Verification items for this drawing (mm, ordinates from the low corner). A direction names the side the tool comes from. Coordinates: 2 decimals unless noted, no trailing zeros. Order: outer loops, then holes, each group sorted by start corner. A loop starts at its lowest first (then second) coordinate and runs counter-clockwise, first axis right, second up. Notation, with made-up numbers: (32, 33) -> (45, 33) arc R20 cw to (45, 68) -> close; hole circle Ø3 at (49.25, -27.5). An arc over 180 degrees is marked (long way). Put each result on its own line as item: value. Start each with the question number.
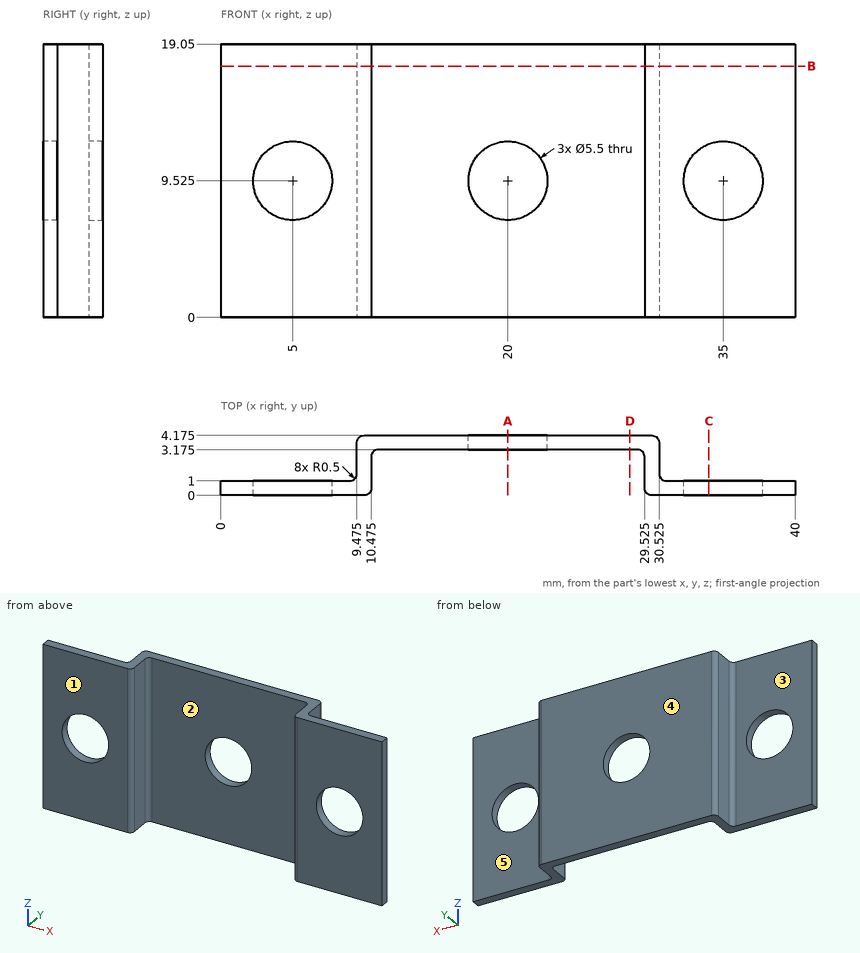
1) Mould release check, pull along X, two halves, no side actions. Record for the marked faces 1 and 2: +X half, -X half, draft (parallel to the pull), parting line (faces both ways), or undercut.
2) Sectioned sample at B-B (z = 17.5). Record the boundary of the cut face in (x, y) (3 decimals).
3) Sectioned sample at C-C (x = 34). Record the boundary of the cut face in (y, z).
4) Gauge pin test, flat ends, axial feed: pin 1 (0.7 mm diameter, centred on y = 2, z = 8, fed in from +X) (3 decimals); pin 2 (4.5 mm diameter, centred on x = 35, z = 9.525, fed in from -Y); pin 3 (2.5 mm diameter, centred on y = 2.5, z = 9.5, fed in from +X); pin 4 (0.7 mm diameter, centred on y = 2.5, z = 7, fed in from -X) (3 decimals). Record the tip position at first contact, or that the pin passes through.
5) Access from +Z, -Z, +X, -X, +Y, -Y to the whole of each face (thin tool, end or side, straight path). Record for the marked faces 3, 4 and 5.
6) Sectioned sample at A-A (x = 20). Record the boundary of the cut face in (y, z) (3 decimals).
7) Sectioned sample at D-D (x = 28.5). Record the boundary of the cut face in (y, z) (3 decimals).
8) Scan lines: line 1 along X through (y, z) = (2.7, 15.5) (3 decimals); line 2 along Z through (x, y) = (35, 0.7) (3 decimals); line 3 along X through (y, z) = (0.5, 9.25) (3 decimals). Record each from-to range of solid material in increasing order. Write a range as [from, to].
Entries:
1. face 1: draft
1. face 2: undercut
2. outline: (0, 0) -> (9.975, 0) arc R0.5 ccw to (10.475, 0.5) -> (10.475, 2.675) arc R0.5 cw to (10.975, 3.175) -> (29.025, 3.175) arc R0.5 cw to (29.525, 2.675) -> (29.525, 0.5) arc R0.5 ccw to (30.025, 0) -> (40, 0) -> (40, 1) -> (31.025, 1) arc R0.5 cw to (30.525, 1.5) -> (30.525, 3.675) arc R0.5 ccw to (30.025, 4.175) -> (9.975, 4.175) arc R0.5 ccw to (9.475, 3.675) -> (9.475, 1.5) arc R0.5 cw to (8.975, 1) -> (0, 1) -> close
3. outline: (0, 0) -> (1, 0) -> (1, 6.96) -> (0, 6.96) -> close; (0, 12.09) -> (1, 12.09) -> (1, 19.05) -> (0, 19.05) -> close
4. pin 1: stops at x = 30.525
4. pin 2: passes through
4. pin 3: stops at x = 30.59
4. pin 4: stops at x = 9.475
5. face 3: +Z, -Z, -X, +Y
5. face 4: +Z, -Z, +X, -X, +Y
5. face 5: +Z, -Z, +X, +Y
6. outline: (3.175, 0) -> (4.175, 0) -> (4.175, 6.775) -> (3.175, 6.775) -> close; (3.175, 12.275) -> (4.175, 12.275) -> (4.175, 19.05) -> (3.175, 19.05) -> close
7. outline: (3.175, 0) -> (4.175, 0) -> (4.175, 19.05) -> (3.175, 19.05) -> close
8. line 1: x = [9.475, 10.476], [29.524, 30.525]
8. line 2: z = [0, 6.775], [12.275, 19.05]
8. line 3: x = [0, 2.264], [7.736, 10.475], [29.525, 32.264], [37.736, 40]
